The listing builds one solid part. Answer for the finished solid, in the listing's coordinates (mm). A direction names the side the tool comes from. Coordinates: 2 decimals unless noted, no trailing zeros. Order: outer loops, then holes, each group sorted by start corner. A loop starts at its lowest first (then second) coordinate and runs counter-clockwise, first axis right, second up. Notation, with made-up numbers: (79.25, 31) -> (118.25, 31) arc R24 ccw to (118.25, 58) -> close; hole circle Ø5 at (44.25, 71). An arc over 180 degrees is marked (long way). Write each question's results on one line, items separated by ' | '. Start each with the question number.
(1) Determine the mould class of faces 4 (the face through (0.596, 2.465, 2.685)), 5 (the face through (0, 2, -11.5)), 6 (the face through (11, -0.012, 24)) for opening direction Z: +Z half, -Z half, draft (parallel to the pull), parting line (faces both ways), or undercut.
(2) Given pin 1 (10 mm diameter, centred on x = -25.5, z = 21.5, fed in from +Y); pin 2 (6.5 mm diameter, centred on x = 0, z = 0, fed in from +Y); pin 3 (15.5 mm diameter, centred on x = -1.5, z = 4, fed in from -Y), each flat-ended and moving along its own axis, determine where each tip first touches the part or whether it passes through.
(3) Straight lines are drawn through the part: L1, parallel to Z at x = 0, y = 2.35; L2, parallel to X at y = 1.5, z = 0; L3, parallel to Z at x = -18.5, y = 4.25. For each, find the intervals that lie inside material, in ascending order.
(4) The part is cut by section A-A, the plane z = 0. Give the vertices of the cut face in (x, y), then the cut area to 4 significant figures.
(5) A tool of negligible diameter and unlimited length cuts with its end or side. For faces 1 (the face through (0, 5, 5)), 2 (the face through (15.5, 2, 5)), 3 (the face through (-15.5, 2, 5)), from which of +Z, -Z, +X, -X, +Y, -Y can it reach the whole face along a straight path? Write none if from no direction.
(6) The part is cut by section D-D, the plane x = 34.5. Give the vertices of the cut face in (y, z).
(7) The part is cut by section B-B, the plane x = 0. Give the vertices of the cut face in (y, z).
(8) The part is cut by section C-C, the plane z = 16. Give the vertices of the cut face in (x, y).
Autodesk Inventor part; units mm, degrees
ref_plane "YZ-Ebene" through (0, 0, 0) normal (1, 0, 0) x (0, 1, 0)
ref_plane "XZ-Ebene" through (0, 0, 0) normal (0, 1, 0) x (-1, 0, 0)
ref_plane "XY-Ebene" through (0, 0, 0) normal (0, 0, 1) x (1, 0, 0)
sketch "Skizze1" plane through (0, 0, 0) normal (0, 1, 0) x (-1, 0, 0)
  line L0 (-15.5, 11.5) -> (15.5, 11.5)
  line L1 (15.5, 11.5) -> (15.5, -11.5)
  line L2 (15.5, -11.5) -> (-15.5, -11.5)
  line L3 (-15.5, -11.5) -> (-15.5, 11.5)
  line L4 (148.7552, 0) -> (-148.7387, 0)
  line L5 (0, -18.1) -> (0, 28.1)
  line L6 (0, -11.5) -> (0, 11.5)
  circle A0 centre (0, 0) radius 2.75
  dimension "d0" = 23
  dimension "d1" = 31
  dimension "d3" = 5.5
extrude "Extrusion1" add sketch "Skizze1" along normal blind 5 contours L0 L5 A0 L4 L3 | L0 L1 L4 A0 L5 | L4 A0 L5 L2 L3 | L1 L2 L5 A0 L4
sketch "Skizze2" plane through (-15.5, 0, 11.5) normal (0, 0, 1) x (1, 0, 0)
  line L0 (0, 0) -> (31, 0)
  line L1 (31, 0) -> (31, 5)
  line L2 (0, 5) -> (31, 5)
  line L3 (0, 0) -> (0, 5)
  line L4 (0, 0) -> (31, 0)
  line L5 (31, 0) -> (31, 5)
  line L6 (0, 5) -> (31, 5)
  line L7 (0, 0) -> (0, 5)
  point P0 (15.5, 0)
extrude "Extrusion2" add sketch "Skizze2" along normal blind 10
sketch "Skizze3" plane through (-15.5, 0, 21.5) normal (0, 0, 1) x (1, 0, 0)
  line L0 (0, 0) -> (31, 0)
  arc A0 (-90.0082, 12.8816) -> (120.9918, 12.8816) centre (15.4918, 1123.4066) ccw
  line L1 (8.3371, 5.988) -> (1.4088, 5.988)
  line L2 (1.4088, 5.988) -> (1.4088, -0.012)
  line L3 (8.3371, -0.012) -> (1.4088, -0.012)
  line L4 (8.3371, 5.988) -> (8.3371, -0.012)
  line L5 (29.5747, 5.988) -> (22.6465, 5.988)
  line L6 (22.6465, 5.988) -> (22.6465, -0.012)
  line L7 (29.5747, -0.012) -> (22.6465, -0.012)
  line L8 (29.5747, 5.988) -> (29.5747, -0.012)
  line L9 (70.4918, 10.8726) -> (70.4918, -5.7752)
  line L10 (-39.5082, 12.8816) -> (-39.5082, -5.1111)
  arc A1 (-39.5082, 7.3287) -> (70.4918, 7.3287) centre (15.4918, 1123.4066) ccw
  arc A2 (-90.7561, 5.0098) -> (121.7396, 5.0098) centre (15.4918, 1123.4066) ccw
  line L11 (8.3371, 5.988) -> (1.4088, 5.988)
  line L12 (1.4088, 5.988) -> (1.4088, -0.012)
  line L13 (8.3371, -0.012) -> (1.4088, -0.012)
  line L14 (8.3371, 5.988) -> (8.3371, -0.012)
  point P0 (15.5, 0)
  point P1 (15.4918, 5.988)
  point P2 (-39.5082, 6.6061)
  point P3 (70.4918, 1.3214)
  point P4 (-39.5082, 1.3214)
  point P5 (7.8951, 0)
  point P6 (22.6465, 0)
  point P7 (29.5747, 0.0626)
  dimension "d9" = 6
  dimension "d10" = 110
extrude "Extrusion3" add sketch "Skizze3" along normal blind 5 contours A2 L2 L1 L4 L0 | A2 L10 A1 L9 L8 L5 L6 L0 L4 L1 L2 | L6 L5 L8 A2 L0 | L0 L8 L7 L6 | A2 L8 L0
properties part number "01-06 Absicherung Box"
Established:
1) face 4: undercut | face 5: -Z half | face 6: draft
2) pin 1: stops at y = 6.39 | pin 2: stops at y = 5 | pin 3: stops at y = 0
3) L1: z = -11.5 to -2.75, 2.75 to 26.5 | L2: x = -15.5 to -2.75, 2.75 to 15.5 | L3: z = 21.5 to 26.5
4) outline: (-15.5, 0) -> (-2.75, 0) -> (-2.75, 5) -> (-15.5, 5) -> close; (2.75, 0) -> (15.5, 0) -> (15.5, 5) -> (2.75, 5) -> close | area: 127.5 mm^2
5) face 1: -Z, +X, -X, +Y | face 2: -Z, +X, +Y, -Y | face 3: -Z, -X, +Y, -Y
6) outline: (0.5, 21.5) -> (6.51, 21.5) -> (6.51, 26.5) -> (0.5, 26.5) -> close
7) outline: (0, -11.5) -> (5, -11.5) -> (5, -2.75) -> (0, -2.75) -> close; (0, 2.75) -> (5, 2.75) -> (5, 21.5) -> (5.97, 21.5) -> (5.97, 26.5) -> (0, 26.5) -> close
8) outline: (-15.5, 0) -> (15.5, 0) -> (15.5, 5) -> (-15.5, 5) -> close
